The drawing under review shows one solid part. Ordinate dimensions are in mm from its lowest x, y, z. Round coordinates to 2 decimals unless told otherwise and drop trailing zeros. Order: outer loops, then holes, each group sorted by start corner. A loop starts at its lowest first (then second) coordinate and runs counter-clockwise, first axis right, second up. Notation, with made-up numbers: M 49,2.5 L 85,2.5 A3 ccw 85,6.5 Z; hole C -31.5,73.25 d5. An arc over 180 degrees is marked long. Answer as a JSON object with one key per item and string values. Group by question number.
1. Add section C-C on z = 2. State the section outline as (x, y) points, and give its area (3 significant figures).
2. To check wall thickness, follow probe 1 along Y at (x, z) = (47.5, 2.1); probe 2 along X at (y, z) = (8, 2.25); probe 3 along Z at (x, y) = (37, 24.5). State the ranges of each line that lie inside material, in increasing order. Write a range as [from, to].
3. Clearance check with flat-ended pins moving along their axes: P1, Ø1.6, axis at y = 17, z = 1, coming from the +X side; P2, Ø12, axis at x = 35, y = 15.5, coming from the -Z side; P3, Ø1.5, axis at x = 43.5, z = 0.5, coming from the +Y side; P4, Ø0.8, axis at x = 29, z = 1, coming from the +Y side. State where each tip first meets the part, or that it passes through.
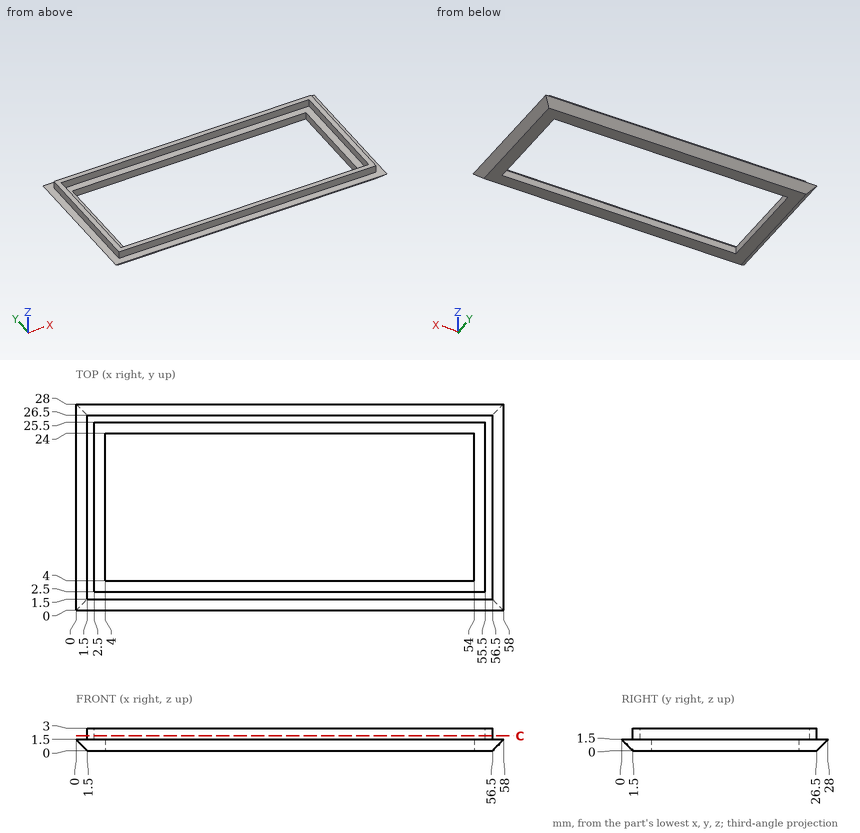
Recorded:
{
 "1": {"outline": "M 1.5,1.5 L 56.5,1.5 L 56.5,26.5 L 1.5,26.5 Z; hole M 2.5,2.5 L 55.5,2.5 L 55.5,25.5 L 2.5,25.5 Z", "area": "156 mm²"},
 "2": {"probe 1": "y = [1.5, 2.5], [25.5, 26.5]", "probe 2": "x = [1.5, 2.5], [55.5, 56.5]", "probe 3": "z = [0, 1.5]"},
 "3": {"P1": "stops at x = 58", "P2": "passes through", "P3": "stops at y = 27.75", "P4": "stops at y = 27.9"}
}
